Build history of the part. All positions in model axes, mm. Face numbers are marked on the shaded views. A direction names the side the tool comes from. Give positions to 0.01 mm unless a question says otherwise; leave off trailing zeros. Write each loop counter-clockwise with the first axis right and the second up, starting at its lowest first coordinate (ties: lowest second). Pieces come first, ordered by that corner, then holes. Notation, with made-up numbers: (12, 42.5) -> (70, 42.5) arc R27 ccw to (70, 71.5) -> close; hole circle Ø7 at (-22, 32). An arc over 180 degrees is marked (long way). Put each result on its own line as item: value.
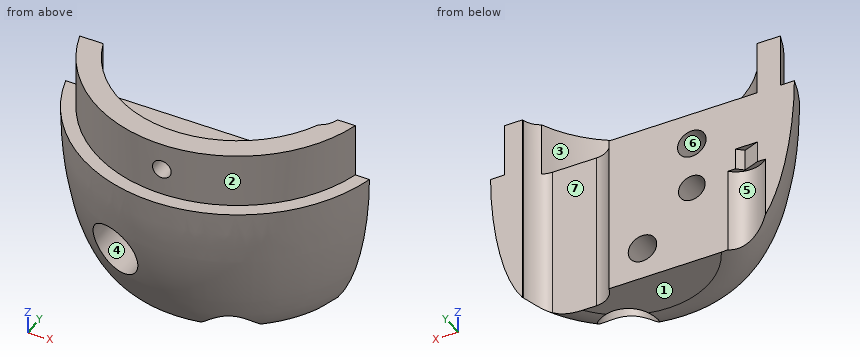
Autodesk Inventor part; units mm, degrees
ref_plane "Work Plane1" through (6.245, 5, -17) normal (0, 0, -1) x (-1, 0, 0)
ref_plane "Work Plane2" through (0, 13.0429, 0) normal (0, 1, 0) x (-1, 0, 0)
ref_plane "YZ Plane" through (0, 0, 0) normal (1, 0, 0) x (0, 1, 0)
sketch "Sketch1" plane through (0, 0, 0) normal (0, 0, 1) x (1, 0, 0)
  point P0 (0, 0)
sketch "Sketch2" plane through (0, 0, 0) normal (1, 0, 0) x (0, 1, 0)
  line L0 (-13.0429, 0) -> (13.0429, 0)
  line L1 (13.0429, 0) -> (13.0429, 3.3095)
  line L2 (13.0429, 3.3095) -> (-13.0429, 3.3095)
  line L3 (-13.0429, 3.3095) -> (-13.0429, 0)
  line L4 (0, 0) -> (0, -15)
  line L5 (0, -15) -> (-8, -15)
  line L6 (-14.2875, 0) -> (14.2875, 0)
  line L7 (14.2875, 0) -> (14.2875, 6.8547)
  line L8 (14.2875, 6.8547) -> (-14.2875, 6.8547)
  line L9 (-14.2875, 6.8547) -> (-14.2875, 0)
  spline S0 degree 4 poles (-14.2875, 0) (-14.2875, -4.9566) (-13.3423, -10.7623) (-11.8115, -15) (-8, -15) knots 0 0 0 0 0 1 1 1 1 1
  point P0 (-12.3627, -11.4481)
  dimension "d1" = 26.0858
  dimension "d2" = 8
  dimension "d3" = 15
  dimension "d4" = 28.575
revolve "Revolution1" add sketch "Sketch2" angle 360 about axis through (0, 0, 0) along (0, 0, -1) contours L0 L4 L5 S0 L6
sketch "Sketch3" plane through (0, 0, 0) normal (0, 0, 1) x (1, 0, 0)
  circle A0 centre (0, 0) radius 14.2875
  circle A1 centre (0, 0) radius 13.0429
  circle A2 centre (0, 0) radius 11
  point P0 (0, -14.2875)
  dimension "d6" = 26.0858
  dimension "d7" = 22
extrude "Extrusion1" add sketch "Sketch3" along normal blind 5 contours A1
hole "Hole1" at (0, 0, 0) direction (0, 0, -1) diameter 3 end through all
sketch "Sketch6" plane through (0, 0, 0) normal (0, 0, 1) x (1, 0, 0)
  circle A0 centre (0, 0) radius 12
  point P0 (4.074, -8.737)
  point P1 (4.82, 8.349)
  point P2 (-9.494, -1.674)
  dimension "d22" = -8.737
  dimension "d23" = 8.349
  dimension "d24" = 1.674
  dimension "d25" = 4.074
  dimension "d26" = 4.82
hole "Hole2" at (-9.494, -1.674, 0) at (4.82, 8.349, 0) at (4.074, -8.737, 0) direction (0, 0, -1) diameter 1.7 end through all
sketch "Sketch8" plane through (0, 0, 0) normal (0, 1, 0) x (-1, 0, 0)
  point P0 (0, 0)
sketch "Sketch9" plane through (0, 0, -15) normal (0, 0, -1) x (-1, 0, 0)
  circle A0 centre (0, 0) radius 1.5
  line L0 (-10.3562, 5) -> (-3, 5)
  line L1 (-3, 5) -> (-3, -5)
  line L2 (-3, -5) -> (-10.3562, -5)
  line L3 (20.0025, 0) -> (-20.0025, 0)
  line L4 (0, -20.0025) -> (0, 20.0025)
  circle A1 centre (-4.82, 8.349) radius 0.85
  circle A2 centre (-4.074, -8.737) radius 0.85
  circle A3 centre (0, 0) radius 8
  arc A4 (-10.3562, 5) -> (-10.3562, -5) centre (0, 0) ccw
  point P0 (0, -8)
  point P1 (-10.7619, 0)
  dimension "d34" = 3
  dimension "d35" = 8.349
  dimension "d36" = 8.737
  dimension "d37" = 10
extrude "Extrusion2" cut sketch "Sketch9" against normal through all contours L3 A3 L0 L1 | L1 L2 A3 L3 | A3 L3 A4 L0 | L2 A4 L3 A3
sketch "Sketch10" plane through (6.245, 5, -15) normal (0, 0, -1) x (-1, 0, 0)
  arc A0 (2.1327, 3.8197) -> (2.1327, 3.8197) centre (2.1327, 3.8197) ccw
  arc A1 (3.0175, -13.6604) -> (3.0175, -13.6604) centre (3.0175, -13.6604) ccw
  arc A2 (16.4746, -6.2481) -> (16.4746, -6.2481) centre (16.4746, -6.2481) ccw
  circle A3 centre (1.425, 3.349) radius 0.85
  circle A4 centre (2.171, -13.737) radius 2.5
  circle A5 centre (2.171, -13.737) radius 0.85
  circle A6 centre (15.739, -6.674) radius 2.5
  circle A7 centre (15.739, -6.674) radius 0.85
  circle A8 centre (1.425, 3.349) radius 2.5
  dimension "d43" = 5
  dimension "d44" = 5
  dimension "d59" = 5
ref_plane "Work Plane1" through (6.245, 5, -17) normal (0, 0, -1) x (-1, 0, 0)
sketch "Sketch11" plane through (6.245, 5, -17) normal (0, 0, -1) x (-1, 0, 0)
  arc A0 (2.1327, 3.8197) -> (2.1327, 3.8197) centre (2.1327, 3.8197) ccw
  arc A1 (16.4746, -6.2481) -> (16.4746, -6.2481) centre (16.4746, -6.2481) ccw
  arc A2 (3.0175, -13.6604) -> (3.0175, -13.6604) centre (3.0175, -13.6604) ccw
  circle A3 centre (1.425, 3.349) radius 2.5
  circle A4 centre (1.425, 3.349) radius 0.85
  circle A5 centre (2.171, -13.737) radius 2.5
  circle A6 centre (15.739, -6.674) radius 2.5
  circle A7 centre (15.739, -6.674) radius 0.85
  circle A8 centre (2.171, -13.737) radius 0.85
  point P0 (6.245, -5)
  dimension "d61" = 5
  dimension "d62" = 5
  dimension "d63" = 5
hole "Hole5" at (4.82, 8.349, -17) at (-9.494, -1.674, -17) at (4.074, -8.737, -17) direction (0, 0, 1) diameter 5 depth 10
sketch "Sketch12" plane through (-9.494, -1.674, -7) normal (0, 0, -1) x (-1, 0, 0)
  circle A0 centre (0, 0) radius 0.85
  circle A1 centre (-14.314, 10.023) radius 0.85
  circle A2 centre (-13.568, -7.063) radius 0.85
  line L0 (-12.264, 8.8394) -> (-14.3141, 7.6559)
  line L1 (-14.3141, 7.6559) -> (-16.364, 8.8395)
  line L2 (-16.364, 8.8395) -> (-16.364, 11.2066)
  line L3 (-16.364, 11.2066) -> (-14.3139, 12.3901)
  line L4 (-14.3139, 12.3901) -> (-12.264, 11.2065)
  line L5 (-12.264, 11.2065) -> (-12.264, 8.8394)
  line L6 (-0.411, -2.3312) -> (-2.2244, -0.8096)
  line L7 (-2.2244, -0.8096) -> (-1.8133, 1.5216)
  line L8 (-1.8133, 1.5216) -> (0.411, 2.3312)
  line L9 (0.411, 2.3312) -> (2.2244, 0.8096)
  line L10 (2.2244, 0.8096) -> (1.8133, -1.5216)
  line L11 (1.8133, -1.5216) -> (-0.411, -2.3312)
  line L12 (-9.494, 1.674) -> (-14.314, 10.023)
  line L13 (-9.494, 1.674) -> (0, 0)
  line L14 (-9.494, 1.674) -> (-13.568, -7.063)
  line L15 (-11.4226, -8.0634) -> (-13.3617, -9.4211)
  line L16 (-13.3617, -9.4211) -> (-15.507, -8.4208)
  line L17 (-15.507, -8.4208) -> (-15.7134, -6.0626)
  line L18 (-15.7134, -6.0626) -> (-13.7743, -4.7049)
  line L19 (-13.7743, -4.7049) -> (-11.629, -5.7052)
  line L20 (-11.629, -5.7052) -> (-11.4226, -8.0634)
  dimension "d71" = 4.1
  dimension "d72" = 4.1
  dimension "d73" = 4.1
extrude "Extrusion3" cut sketch "Sketch12" against normal blind 2 contours L7 L8 L9 L10 L11 L6 | A2 | L19 L20 L15 L16 L17 L18 | L0 L1 L2 L3 L4 L5
ref_plane "Work Plane2" through (0, 13.0429, 0) normal (0, 1, 0) x (-1, 0, 0)
sketch "Sketch13" plane through (0, 13.0429, 0) normal (0, 1, 0) x (-1, 0, 0)
  line L0 (-13.0429, 5) -> (13.0429, 5)
  line L1 (-13.0429, 0) -> (13.0429, 0)
  line L2 (0, -19.0003) -> (0, 9.0001)
  point P0 (0, 0)
  point P1 (0, 2.5)
  dimension "d76" = 2.5
hole "Hole6" at (0, 13.0429, 2.5) direction (0, -1, 0) diameter 1.694 end through all
ref_plane "Work Plane3" through (0, -3.5, 0) normal (0, 1, 0) x (-1, 0, 0)
fillet "Fillet1" radius 2 4 edges at (3, -5, -7.5) (3, 5, -7.5) (10.3562, 5, -4.0051) (10.3562, -5, -4.0051)
sketch "Sketch14" plane through (0, -3.5, 0) normal (0, 1, 0) x (-1, 0, 0)
  line L0 (-22.1309, 11.369) -> (21.5238, 11.369)
  line L1 (21.5238, 11.369) -> (21.5238, -19.3162)
  line L2 (21.5238, -19.3162) -> (-22.1309, -19.3162)
  line L3 (-22.1309, -19.3162) -> (-22.1309, 11.369)
  point P0 (0, 0)
extrude "Extrusion4" cut sketch "Sketch14" along normal through all
sketch "Sketch15" plane through (0, -3.5, 0) normal (0, 1, 0) x (1, 0, 0)
  line L0 (3.0635, 0) -> (-10.4283, 0)
  line L1 (-7.1937, 15) -> (3.0635, 15)
  line L2 (0, 19.0003) -> (0, -9.0001)
  circle A0 centre (-4.5, 3) radius 1.3
  circle A1 centre (0, 12) radius 1.3
  point P0 (0, 0)
  point P1 (-4.5, 7.5)
  dimension "d88" = 3
  dimension "d89" = 4.5
  dimension "d90" = 4.5
  dimension "d91" = 7.5
  dimension "d92" = 3
  dimension "d93" = 2.6
  dimension "d94" = 2.6
extrude "Extrusion5" cut sketch "Sketch15" against normal blind 3.2
hole "Hole7" at (-4.5, -3.5, -7.5) direction (0, -1, 0) diameter 2.438 end through all
ref_plane "Work Plane4" through (0, -14.5, 0) normal (0, -1, 0) x (1, 0, 0)
sketch "Sketch16" plane through (0, -14.5, 0) normal (0, -1, 0) x (1, 0, 0)
  point P0 (0, 0)
sketch "Sketch17" plane through (0, -14.5, 0) normal (0, -1, 0) x (1, 0, 0)
  arc A0 (-5.6245, -7.9706) -> (-5.6245, -7.9706) centre (-5.6245, -7.9706) ccw
  point P0 (0, 0)
  point P1 (-4.5, -7.5)
hole "Hole8" at (-4.5, -14.5, -7.5) direction (0, 1, 0) diameter 5 depth 8
properties part number "Handle_2_Back_Bottom"
1) Pin check, flat tips, straight feed: pin 1 (10 mm diameter, centred on x = 6.5, z = -4.5, fed in from -Y); pin 2 (4.5 mm diameter, centred on x = -4.5, z = -7.5, fed in from -Y); pin 3 (2 mm diameter, centred on x = 10, z = -10.5, fed in from -Y). Stop position of each tip, or through.
Filled sheet:
pin 1: y = -14.07
pin 2: y = -6.5
pin 3: y = -9.13
2) Slice it at B-B (z = -7.5). Give the number of separate pieces and of enclosed holes in the cut face, plus the area to 3 significant figures.
Filled sheet:
separate pieces: 2
enclosed holes: 1
area: 125 mm2
3) Wall check: L1, parallel to Z at x = -4.5, y = -4.6; L2, parallel to X at y = -10.25, z = -10.25; L3, parallel to Z at x = -5, y = -4.25. Give the ranges that are in metal, low to high.
Filled sheet:
L1: -15 to -8.72, -6.28 to -4.3, -1.7 to 0
L2: -7.71 to 2.08, 6.06 to 7.71
L3: -15 to -8.61, -6.39 to -4.2, -1.8 to 0
4) Tool access for the marked faces 4, 5, 6 and 7: list every direction of +Z, -Z, +X, -X, +Y, -Y with a clear straight run to the whole face (end or side of a thin tool).
Filled sheet:
face 4: -Y
face 5: -Z, +Y
face 6: +Y
face 7: +Z, -Z, +Y
5) Slice it at A-A (z = 2.5). Write the cut outline in (x, y).
Filled sheet:
outline: (-12.56, -3.5) arc R13.04 ccw to (-0.85, -13.02) -> (-0.85, -10.97) arc R11 cw to (-10.43, -3.5) -> close; (0.85, -13.02) arc R13.04 ccw to (12.56, -3.5) -> (10.95, -3.5) arc R11.5 cw to (10.91, -3.63) arc R2 cw to (9.9, -4.79) arc R11 cw to (0.85, -10.97) -> close
6) Pull direction X, two halves, no side cores. Call the marked faces 1, 2 and 3: released by +X, released by -X, zero draft, split by the parting line, or undercut.
Filled sheet:
face 1: zero draft
face 2: split by the parting line
face 3: undercut
